Build history of the part. All positions in model axes, mm. Face numbers are marked on the shaded views. A direction names the side the tool comes from. Round coordinates to 2 decimals unless told otherwise and drop trailing zeros. Write each loop counter-clockwise with the first axis right and the second up, starting at its lowest first coordinate (ties: lowest second). Pieces come first, ordered by that corner, then holes. Notation, with made-up numbers: (61.5, 79.5) - (112.5, 79.5) arc R13 ccw to (112.5, 85.5) - close; hole circle Ø6 at (-24, 67.25). An arc over 180 degrees is marked (long way). Answer as a JSON object with one key per item and string values. Group by question number.
Item 1: Which spindle directions (+Z, -Z, +X, -X, +Y, -Y) get a long thin tool onto all of the face, cutting with end or side? Do the marked faces 5, 6 and 7. Say none if no direction does.
Item 2: Slice it at A-A, the plane z = 0.5. List the corners of the cut face in (x, y).
Item 3: Slice it at B-B, the plane y = 2.25. List the corners of the cut face in (x, z).
Item 4: Two-plate mould, pull along Y, no slides. Class the marked faces 1, 2, 3 and 4: +Y half, -Y half, draft (parallel to the pull), parting line (faces both ways), or undercut.
Item 5: Probe line 1 (X direction, y = 0, z = 0.75); line 2 (X direction, y = 1.5, z = 1.55). List the from-to ranges inside material, lowest first. Write a range as from..to.
Item 6: Flat gauge pins, fed straight in: pin 1 (1 mm diameter, centred on x = -1, z = 0.5, fed in from +Y); pin 2 (1 mm diameter, centred on x = 2, z = 1.5, fed in from +Y); pin 3 (0.6 mm diameter, centred on x = 2, y = 4.5, fed in from +Z). Where does each tip first touch, or does it go through?
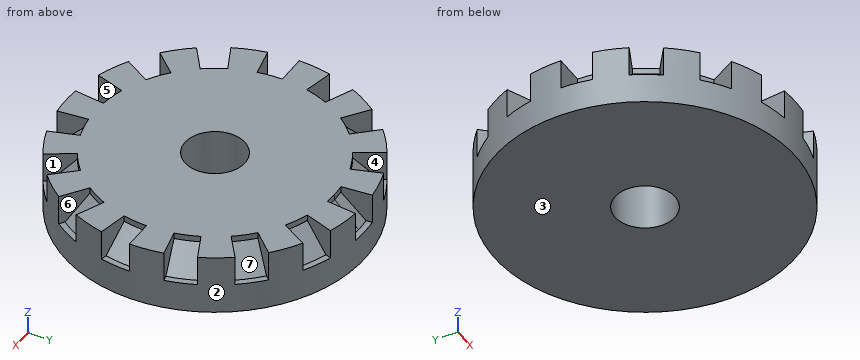
from build123d import *

# Parameters (mm, degrees)
F0_W     = 4
F0_H     = 2
F3_DEPTH = 1
F4_SIZE  = 0.8


with BuildPart() as f1:
    # F0 (on Front) → F1 (revolve)
    with BuildSketch(Plane.XZ):
        with Locations((-3, 1)):
            Rectangle(F0_W, F0_H)
    revolve(axis=Axis((0, 0, 1), (0, 0, 1)))

    # F2 (on face) → F3 (cut)
    with BuildSketch(Plane.XY.offset(2)):
        with BuildLine():
            ThreePointArc((-0.4, 3.9799497484), (-0.2002511002, 3.9949842924), (0, 4))
            Line((0, 4), (0, 4.9749371855))
            Line((0, 4.9749371855), (-0.5, 4.9749371855))
            Line((-0.5, 4.9749371855), (-0.4, 3.9799497484))
        make_face()
        with BuildLine():
            Line((0, 4.9749371855), (0, 4))
            ThreePointArc((0, 4), (0.2002511002, 3.9949842924), (0.4, 3.9799497484))
            Line((0.4, 3.9799497484), (0.5, 4.9749371855))
            Line((0.5, 4.9749371855), (0, 4.9749371855))
        make_face()
        with BuildLine():
            Line((0, 5), (0, 4.9749371855))
            Line((0, 4.9749371855), (0.5, 4.9749371855))
            ThreePointArc((0.5, 4.9749371855), (0.2503138753, 4.9937303656), (0, 5))
        make_face()
        with BuildLine():
            Line((-0.5, 4.9749371855), (0, 4.9749371855))
            Line((0, 4.9749371855), (0, 5))
            ThreePointArc((0, 5), (-0.2503138753, 4.9937303656), (-0.5, 4.9749371855))
        make_face()
        with BuildLine():
            Line((1.5667165215, 4.7481995894), (1.2533732172, 3.7985596716))
            ThreePointArc((1.2533732172, 3.7985596716), (1.6269465723, 3.6541818306), (1.9842095833, 3.4731703571))
            Line((1.9842095833, 3.4731703571), (2.4802619792, 4.3414629464))
            ThreePointArc((2.4802619792, 4.3414629464), (2.0336832154, 4.5677272882), (1.5667165215, 4.7481995894))
        make_face()
        with BuildLine():
            Line((3.3625335233, 3.7004551483), (2.6900268187, 2.9603641186))
            ThreePointArc((2.6900268187, 2.9603641186), (2.9725793019, 2.6765224254), (3.2253313037, 2.3658482583))
            Line((3.2253313037, 2.3658482583), (4.0316641297, 2.9573103228))
            ThreePointArc((4.0316641297, 2.9573103228), (3.7157241274, 3.3456530318), (3.3625335233, 3.7004551483))
        make_face()
        with BuildLine():
            Line((4.5769379313, 2.0128683944), (3.661550345, 1.6102947155))
            ThreePointArc((3.661550345, 1.6102947155), (3.8042260652, 1.2360679775), (3.9087639405, 0.8494495025))
            Line((3.9087639405, 0.8494495025), (4.8859549256, 1.0618118781))
            ThreePointArc((4.8859549256, 1.0618118781), (4.7552825815, 1.5450849719), (4.5769379313, 2.0128683944))
        make_face()
        with BuildLine():
            Line((4.9999481907, -0.0227615912), (3.9999585526, -0.0182092729))
            ThreePointArc((3.9999585526, -0.0182092729), (3.9780875815, -0.4181138531), (3.916335782, -0.8138267892))
            Line((3.916335782, -0.8138267892), (4.8954197275, -1.0172834865))
            ThreePointArc((4.8954197275, -1.0172834865), (4.9726094768, -0.5226423163), (4.9999481907, -0.0227615912))
        make_face()
        with BuildLine():
            Line((4.5584219849, -2.0544558909), (3.6467375879, -1.6435647127))
            ThreePointArc((3.6467375879, -1.6435647127), (3.4641016151, -2), (3.2467375879, -2.3363850357))
            Line((3.2467375879, -2.3363850357), (4.0584219849, -2.9204812947))
            ThreePointArc((4.0584219849, -2.9204812947), (4.3301270189, -2.5), (4.5584219849, -2.0544558909))
        make_face()
        with BuildLine():
            Line((3.3287032059, -3.7309161029), (2.6629625647, -2.9847328823))
            ThreePointArc((2.6629625647, -2.9847328823), (2.3511410092, -3.2360679775), (2.0157489692, -3.4549610842))
            Line((2.0157489692, -3.4549610842), (2.5196862116, -4.3187013552))
            ThreePointArc((2.5196862116, -4.3187013552), (2.9389262615, -4.0450849719), (3.3287032059, -3.7309161029))
        make_face()
        with BuildLine():
            Line((1.5234214023, -4.7622670264), (1.2187371219, -3.8098136211))
            ThreePointArc((1.2187371219, -3.8098136211), (0.8316467633, -3.9125904029), (0.4362190413, -3.9761429738))
            Line((0.4362190413, -3.9761429738), (0.5452738016, -4.9701787172))
            ThreePointArc((0.5452738016, -4.9701787172), (1.0395584541, -4.8907380037), (1.5234214023, -4.7622670264))
        make_face()
        with BuildLine():
            Line((-0.5452738016, -4.9701787172), (-0.4362190413, -3.9761429738))
            ThreePointArc((-0.4362190413, -3.9761429738), (-0.8316467633, -3.9125904029), (-1.2187371219, -3.8098136211))
            Line((-1.2187371219, -3.8098136211), (-1.5234214023, -4.7622670264))
            ThreePointArc((-1.5234214023, -4.7622670264), (-1.0395584541, -4.8907380037), (-0.5452738016, -4.9701787172))
        make_face()
        with BuildLine():
            Line((-2.5196862116, -4.3187013552), (-2.0157489692, -3.4549610842))
            ThreePointArc((-2.0157489692, -3.4549610842), (-2.3511410092, -3.2360679775), (-2.6629625647, -2.9847328823))
            Line((-2.6629625647, -2.9847328823), (-3.3287032059, -3.7309161029))
            ThreePointArc((-3.3287032059, -3.7309161029), (-2.9389262615, -4.0450849719), (-2.5196862116, -4.3187013552))
        make_face()
        with BuildLine():
            Line((-4.0584219849, -2.9204812947), (-3.2467375879, -2.3363850357))
            ThreePointArc((-3.2467375879, -2.3363850357), (-3.4641016151, -2), (-3.6467375879, -1.6435647127))
            Line((-3.6467375879, -1.6435647127), (-4.5584219849, -2.0544558909))
            ThreePointArc((-4.5584219849, -2.0544558909), (-4.3301270189, -2.5), (-4.0584219849, -2.9204812947))
        make_face()
        with BuildLine():
            Line((-4.8954197275, -1.0172834865), (-3.916335782, -0.8138267892))
            ThreePointArc((-3.916335782, -0.8138267892), (-3.9780875815, -0.4181138531), (-3.9999585526, -0.0182092729))
            Line((-3.9999585526, -0.0182092729), (-4.9999481907, -0.0227615912))
            ThreePointArc((-4.9999481907, -0.0227615912), (-4.9726094768, -0.5226423163), (-4.8954197275, -1.0172834865))
        make_face()
        with BuildLine():
            Line((-4.8859549256, 1.0618118781), (-3.9087639405, 0.8494495025))
            ThreePointArc((-3.9087639405, 0.8494495025), (-3.8042260652, 1.2360679775), (-3.661550345, 1.6102947155))
            Line((-3.661550345, 1.6102947155), (-4.5769379313, 2.0128683944))
            ThreePointArc((-4.5769379313, 2.0128683944), (-4.7552825815, 1.5450849719), (-4.8859549256, 1.0618118781))
        make_face()
        with BuildLine():
            Line((-4.0316641297, 2.9573103228), (-3.2253313037, 2.3658482583))
            ThreePointArc((-3.2253313037, 2.3658482583), (-2.9725793019, 2.6765224254), (-2.6900268187, 2.9603641186))
            Line((-2.6900268187, 2.9603641186), (-3.3625335233, 3.7004551483))
            ThreePointArc((-3.3625335233, 3.7004551483), (-3.7157241274, 3.3456530318), (-4.0316641297, 2.9573103228))
        make_face()
        with BuildLine():
            Line((-2.4802619792, 4.3414629464), (-1.9842095833, 3.4731703571))
            ThreePointArc((-1.9842095833, 3.4731703571), (-1.6269465723, 3.6541818306), (-1.2533732172, 3.7985596716))
            Line((-1.2533732172, 3.7985596716), (-1.5667165215, 4.7481995894))
            ThreePointArc((-1.5667165215, 4.7481995894), (-2.0336832154, 4.5677272882), (-2.4802619792, 4.3414629464))
        make_face()
    extrude(amount=-F3_DEPTH, mode=Mode.SUBTRACT)

    # F4
    f4_edges = [f1.edges().sort_by_distance(p)[0] for p in [
        (-3.978088, -0.418114, 1),
        (-3.464102, -2, 1),
        (-2.351141, -3.236068, 1),
        (-0.831647, -3.91259, 1),
        (0.831647, -3.91259, 1),
        (2.351141, -3.236068, 1),
        (3.464102, -2, 1),
        (3.978088, -0.418114, 1),
        (3.804226, 1.236068, 1),
        (2.972579, 2.676522, 1),
        (1.626947, 3.654182, 1),
        (0, 4, 1),
        (-1.626947, 3.654182, 1),
        (-2.972579, 2.676522, 1),
        (-3.804226, 1.236068, 1),
    ]]
    chamfer(f4_edges, length=F4_SIZE)


solid = f1.part
Geometry says:
{
 "1": {"face 5": "+Z, -Y", "face 6": "+Z, +X", "face 7": "+Z"},
 "2": {"outline": "circle Ø10 at (0, 0); hole circle Ø2 at (0, 0)"},
 "3": {"outline": "(-4.47, 0) - (4.47, 0) - (4.47, 2) - (-4.47, 2) - close"},
 "4": {"face 1": "undercut", "face 2": "parting line", "face 3": "draft", "face 4": "+Y half"},
 "5": {"line 1": "x = -5..-1, 1..5", "line 2": "x = -3.98..3.98"},
 "6": {"pin 1": "stops at y = 4.97", "pin 2": "stops at y = 4.77", "pin 3": "stops at z = 1.18"}
}
